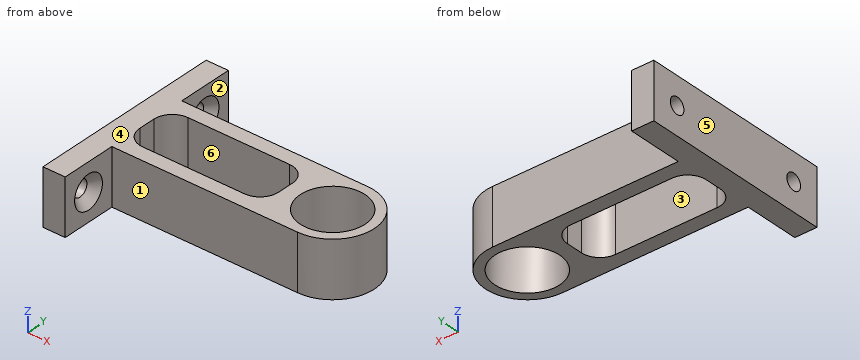
from build123d import *

# Parameters (mm, degrees)
F0_R                 = 8.75
F1_DEPTH             = 15
F4_D                 = 4.4
F4_CSINK_D           = 8.96
F4_CSINK_ANGLE       = 90
F4_ON_F3_D           = 4.4
F4_ON_F3_CSINK_D     = 8.96
F4_ON_F3_CSINK_ANGLE = 90
F5_W                 = 37.5
F5_H                 = 14.5
F6_DEPTH             = 25
F7_R                 = 5


with BuildPart() as f1:
    # F0 (on Top) → F1 (new body)
    with BuildSketch(Plane.XY):
        with BuildLine():
            Line((-50.25, -11.25), (0, -11.25))
            ThreePointArc((0, -11.25), (11.25, 0), (0, 11.25))
            Line((0, 11.25), (-50.25, 11.25))
            Line((-50.25, 11.25), (-50.25, 26.25))
            Line((-50.25, 26.25), (-56.25, 26.25))
            Line((-56.25, 26.25), (-56.25, -26.25))
            Line((-56.25, -26.25), (-50.25, -26.25))
            Line((-50.25, -26.25), (-50.25, -11.25))
        make_face()
        Circle(F0_R, mode=Mode.SUBTRACT)
    extrude(amount=F1_DEPTH)

    # F4 (through all)
    with Locations(Plane.YZ.offset(-50.25)):
        with Locations((-18.75, 7.5)):
            CounterSinkHole(F4_D / 2, F4_CSINK_D / 2, counter_sink_angle=F4_CSINK_ANGLE)

    # F4 on F3 (through all)
    with Locations(Plane.YZ.offset(-50.25)):
        with Locations((18.75, 7.5)):
            CounterSinkHole(F4_ON_F3_D / 2, F4_ON_F3_CSINK_D / 2, counter_sink_angle=F4_ON_F3_CSINK_ANGLE)

    # F5 (on face) → F6 (cut)
    with BuildSketch(Plane.XY.offset(15)):
        with Locations((-31.5, 0)):
            Rectangle(F5_W, F5_H)
    extrude(amount=-F6_DEPTH, mode=Mode.SUBTRACT)

    # F7
    f7_edges = [f1.edges().sort_by_distance(p)[0] for p in [
        (-50.25, 7.25, 7.5),
        (-50.25, -7.25, 7.5),
        (-12.75, 7.25, 7.5),
        (-12.75, -7.25, 7.5),
    ]]
    fillet(f7_edges, radius=F7_R)


solid = f1.part
Work out the finished part from the listing and answer in its coordinate system (mm). Face numbers are marked on the shaded views. A direction names the side the tool comes from. Round coordinates to 2 decimals unless told otherwise and drop trailing zeros. Order: outer loops, then holes, each group sorted by start corner. A loop starts at its lowest first (then second) coordinate and runs counter-clockwise, first axis right, second up. Notation, with made-up numbers: M 34,43.25 L 76,43.25 A18 cw 76,47.25 Z; hole C 81.5,84.5 d4. An arc over 180 degrees is marked long. Put each result on its own line as item: value. Start each with the question number.
Q1. Section B-B, the plane y = 18.75 is taken. Write down the section's boundary in (x, z).
Q2. Flat-ended cylindrical pins translate along their axes: pin 1 (4.5 mm diameter, centred on y = -18, z = 8.5, fed in from +X); pin 2 (1 mm diameter, centred on x = -33.5, z = 11, fed in from +Y); pin 3 (3.5 mm diameter, centred on y = -18.75, z = 7.5, fed in from +X); pin 4 (1 mm diameter, centred on y = -7.5, z = 8.5, fed in from +X). Find the tip coordinate at first contact, or state that the pin passes through.
Q3. For a pull along X with two mould halves and no side action, classify the marked faces 4, 5 and 6 as pulls with the +X half, pulls with the -X half, needs draft (parallel to the pull), parting line crosses it, or undercut.
Q4. A tool of negligible diameter and unlimited length cuts with its end or side. For the marked faces 1, 2 and 3, from which of +Z, -Z, +X, -X, +Y, -Y can it reach the whole face along a straight path? Write none if from no direction.
Q5. Straight lines are drawn through the part: L1, parallel to Y at x = -53.95, z = 7.5; L2, parallel to Y at x = -35, z = 6.5; L3, parallel to Z at x = -53.25, y = 18.75. For each, find the intervals that lie inside material, in ascending order. Write a range as [from, to].
Q6. Section D-D, the plane z = 1 is taken. Write down the section's boundary in (x, y).
Q7. Section A-A, the plane z = 7.5 is taken. Give the number of separate pieces and of enclosed holes in the cut face, and give its area (3 significant figures).
Q8. Section C-C, the plane x = -51 is taken. Write down the section's boundary in (y, z), and give its area (3 significant figures).
Findings below:
1. outline: M -56.25,0 L -50.25,0 L -50.25,3.02 L -52.53,5.3 L -56.25,5.3 Z; M -56.25,9.7 L -52.53,9.7 L -50.25,11.98 L -50.25,15 L -56.25,15 Z
2. pin 1: stops at x = -51.23
2. pin 2: stops at y = 11.25
2. pin 3: passes through
2. pin 4: stops at x = 8.81
3. face 4: needs draft
3. face 5: pulls with the -X half
3. face 6: undercut
4. face 1: +Z, -Z, +X, -Y
4. face 2: +Z, -Z, +X, +Y
4. face 3: +Z, -Z
5. L1: y = [-26.25, -20.95], [-16.55, 16.55], [20.95, 26.25]
5. L2: y = [-11.25, -7.25], [7.25, 11.25]
5. L3: z = [0, 5.3], [9.7, 15]
6. outline: M -56.25,-26.25 L -50.25,-26.25 L -50.25,-11.25 L 0,-11.25 A11.25 ccw 0,11.25 L -50.25,11.25 L -50.25,26.25 L -56.25,26.25 Z; hole M -50.25,-2.25 A5 ccw -45.25,-7.25 L -17.75,-7.25 A5 ccw -12.75,-2.25 L -12.75,2.25 A5 ccw -17.75,7.25 L -45.25,7.25 A5 ccw -50.25,2.25 Z; hole C 0,0 d17.5
7. separate pieces: 3
7. enclosed holes: 2
7. area: 818 mm^2
8. outline: M -26.25,0 L 26.25,0 L 26.25,15 L -26.25,15 Z; hole C -18.75,7.5 d7.46; hole C 18.75,7.5 d7.46
8. area: 700 mm^2
